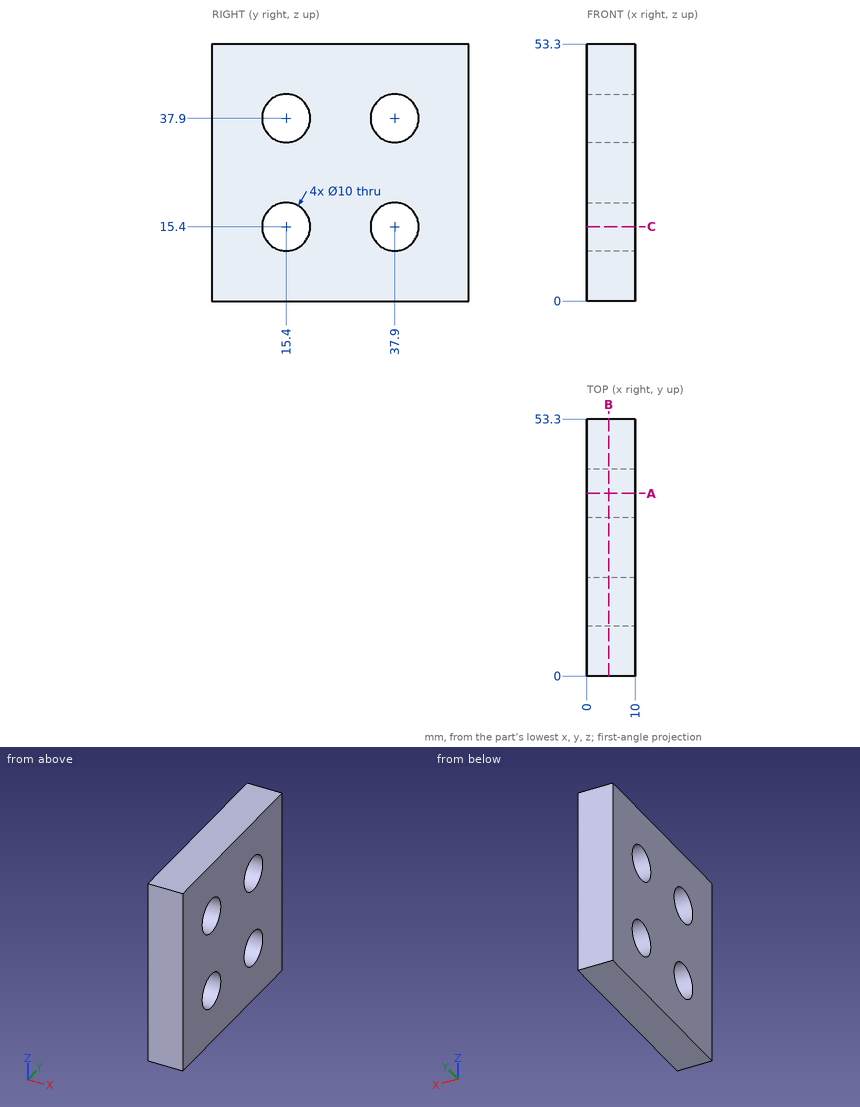
The figure shows three views and two pictorial views of one solid part (mm, origin at its lowest corner). Answer the questions. Coordinates: 2 decimals unless noted, no trailing zeros. Loops run counter-clockwise (first coordinate to the right, second up) from the corner with the lowest first, then second, coordinate; pieces in that order, holes last.
1) A flat-ended cylindrical pin translates along its axis: pin 1 Ø8 at (y, z) = (15.4, 15.4) entering from +X. Find the tip coordinate at first contact, or state that the pin passes through.
2) Find the intervals of material crossed by L1, parallel to Z at x = 8, y = 37.9; L2, parallel to Y at x = 4.5, z = 40.5; L3, parallel to Z at x = 3.25, y = 13, in increasing order.
3) Find section A-A on y = 37.9. Write down the section's boundary in (x, z).
4) Find section B-B on x = 4.5. Write down the section's boundary in (y, z), then the cut area to 3 significant figures.
Values:
1. pin 1: passes through
2. L1: z = 0 to 10.4, 20.4 to 32.9, 42.9 to 53.3
2. L2: y = 0 to 11.13, 19.67 to 33.63, 42.17 to 53.3
2. L3: z = 0 to 11.01, 19.79 to 33.51, 42.29 to 53.3
3. outline: (0, 0) - (10, 0) - (10, 10.4) - (0, 10.4) - close; (0, 20.4) - (10, 20.4) - (10, 32.9) - (0, 32.9) - close; (0, 42.9) - (10, 42.9) - (10, 53.3) - (0, 53.3) - close
4. outline: (0, 0) - (53.3, 0) - (53.3, 53.3) - (0, 53.3) - close; hole circle Ø10 at (15.4, 15.4); hole circle Ø10 at (15.4, 37.9); hole circle Ø10 at (37.9, 15.4); hole circle Ø10 at (37.9, 37.9)
4. area: 2,530 mm2
